Work out the finished part from the listing and answer in its coordinate system (mm). A direction names the side the tool comes from. Round coordinates to 2 decimals unless told otherwise and drop trailing zeros. Loops run counter-clockwise (first coordinate to the right, second up) from the corner with the lowest first, then second, coordinate; pieces in that order, holes last. Notation, with made-up numbers: (15.25, -39.75) - (34.25, -39.75) arc R30 cw to (34.25, -4.75) - close; hole circle Ø4 at (37, 60.5). An arc over 180 degrees is marked (long way). Return JSON: item names as keys, results as strings.
Autodesk Inventor part; units mm, degrees
ref_plane "YZ Plane" through (0, 0, 0) normal (1, 0, 0) x (0, 1, 0)
ref_plane "XZ Plane" through (0, 0, 0) normal (0, 1, 0) x (-1, 0, 0)
ref_plane "XY Plane" through (0, 0, 0) normal (0, 0, 1) x (1, 0, 0)
sketch "Skizze1" plane through (0, 0, 0) normal (0, 0, 1) x (1, 0, 0)
  line L0 (0, -2.4) -> (0, 14.4)
  line L1 (-30.1, 0) -> (30.1, 0)
  arc A0 (21.5, 10.5) -> (18.5, 10.5) centre (20, 10.5) ccw
  line L2 (21.5, 10.5) -> (21.5, 8)
  line L3 (21.5, 8) -> (-21.5, 8)
  line L4 (-21.5, 8) -> (-21.5, 10)
  line L5 (-21.5, 10) -> (-16.7, 10)
  line L6 (-16.7, 10) -> (-16.7, 10.5)
  line L7 (-16.7, 10.5) -> (18.5, 10.5)
  point P0 (0, 0)
  dimension "d0" = 3
  dimension "d1" = 21
  dimension "d2" = 16
  dimension "d3" = 43
  dimension "d4" = 4.8
  dimension "d5" = 20
revolve "Umdrehung1" add sketch "Skizze1" angle 360 about axis through (-10, 0, 0) along (1, 0, 0)
properties part number "Zylinder"
1) A tool of negligible diameter and unlimited length cuts with its end or side. For faces 4 (the flat face through (-21.5, 0, 8.2)), 5 (the cylindrical face through (-19.07, -2.17, -9.76)), from which of +Z, -Z, +X, -X, +Y, -Y can it reach the whole face along a straight path? Write none if from no direction.
Verdict:
{"face 4": "+Z, -Z, -X, +Y, -Y", "face 5": "-X"}
2) Section A-A (z = 0) is taken. Give the vertices of the cut face in (x, y).
Verdict:
{"outline": "(-21.5, -10) - (-16.7, -10) - (-16.7, -10.5) - (18.5, -10.5) arc R1.5 ccw to (21.5, -10.5) - (21.5, -8) - (-21.5, -8) - close; (-21.5, 8) - (21.5, 8) - (21.5, 10.5) arc R1.5 ccw to (18.5, 10.5) - (-16.7, 10.5) - (-16.7, 10) - (-21.5, 10) - close"}
3) Flat-ended cylindrical pins translate along their axes: pin 1 (8 mm diameter, centred on x = -1.5, z = -5.5, fed in from +Y); pin 2 (3 mm diameter, centred on x = 12.5, y = 4.5, fed in from -Z); pin 3 (6.5 mm diameter, centred on y = -2, z = 0, fed in from -X); pin 4 (5 mm diameter, centred on x = 14.5, y = -8.5, fed in from +Z). Find the tip coordinate at first contact, or state that the pin passes through.
Verdict:
{"pin 1": "stops at y = 10.39", "pin 2": "stops at z = -10.06", "pin 3": "passes through", "pin 4": "stops at z = 8.62"}
4) Find the intervals of material crossed by L1, parallel to Z at x = -4, y = 0; L2, parallel to X at y = -9, z = -5.5; L3, parallel to Z at x = 7.5, y = 6.75, in increasing order.
Verdict:
{"L1": "z = -10.5 to -8, 8 to 10.5", "L2": "x = 18.5 to 21.5", "L3": "z = -8.04 to -4.29, 4.29 to 8.04"}
5) Section C-C (x = 16) is taken. Give the vertices of the cut face in (y, z), and give its area (3 significant figures).
Verdict:
{"outline": "circle Ø21 at (0, 0); hole circle Ø16 at (0, 0)", "area": "145 mm2"}
6) Determine the mould class of faces 1 (the cylindrical face through (1.1, 10, 3.2)), 2 (the flat face through (-16.7, 5, -9)), 3 (the cylindrical face through (-0.3, -1.73, 7.81)) for opening direction Y: pulls with the +Y half, pulls with the -Y half, needs draft (parallel to the pull), parting line crosses it, or undercut.
Verdict:
{"face 1": "parting line crosses it", "face 2": "needs draft", "face 3": "undercut"}
